Check sheet for the drawn part. Datum: minimum x, y, z corner. Units: mm. A direction names the side the tool comes from. Coordinates: 2 decimals unless noted, no trailing zeros. Write each loop counter-clockwise with the first axis right and the second up, starting at its lowest first coordinate (ties: lowest second). Pieces come first, ordered by that corner, then holes. Notation, with made-up numbers: (89.25, 45.5) -> (128.25, 45.5) arc R6 cw to (128.25, 52.5) -> close; hole circle Ø11 at (71, 89). An arc over 180 degrees is marked (long way). Answer in a Markdown table with one row per item. Add a question column.
Q1. Section check A-A, the plane x = 5. Record the boundary of the cut face in (y, z), and give its area (3 significant figures).
Q2. Section check B-B, the plane y = 15.25. Record the boundary of the cut face in (x, z).
Q3. Section check C-C, the plane z = 5. Record the boundary of the cut face in (x, y), and give its area (3 significant figures).
Q4. Gauge pin test, flat ends, axial feed: P1, Ø4, axis at x = 5, z = 5, coming from the +Y side; P2, Ø1.5, axis at y = 17, z = 15, coming from the +X side; P3, Ø1, axis at y = 14.5, z = 45.5, coming from the +X side; P4, Ø10, axis at x = 38.5, y = 6.5, coming from the +Z side. Record the tip position at first contact, or that the pin passes through.
Q5. Section check D-D, the plane x = 27.5. Record the boundary of the cut face in (y, z).
Q6. Tool access check on the marked faces 1 and 2. Record the directions out of +Z, -Z, +X, -X, +Y, -Y that give a thin tool (end or side, any length) a straight path to the whole face; none if there is none.
Q7. Thickness scan on line 1 (X direction, y = 10.75, z = 33); line 2 (Z direction, x = 39.5, y = 5.5); line 3 (X direction, y = 19.5, z = 5). Record the ranges inside material, lowest first.
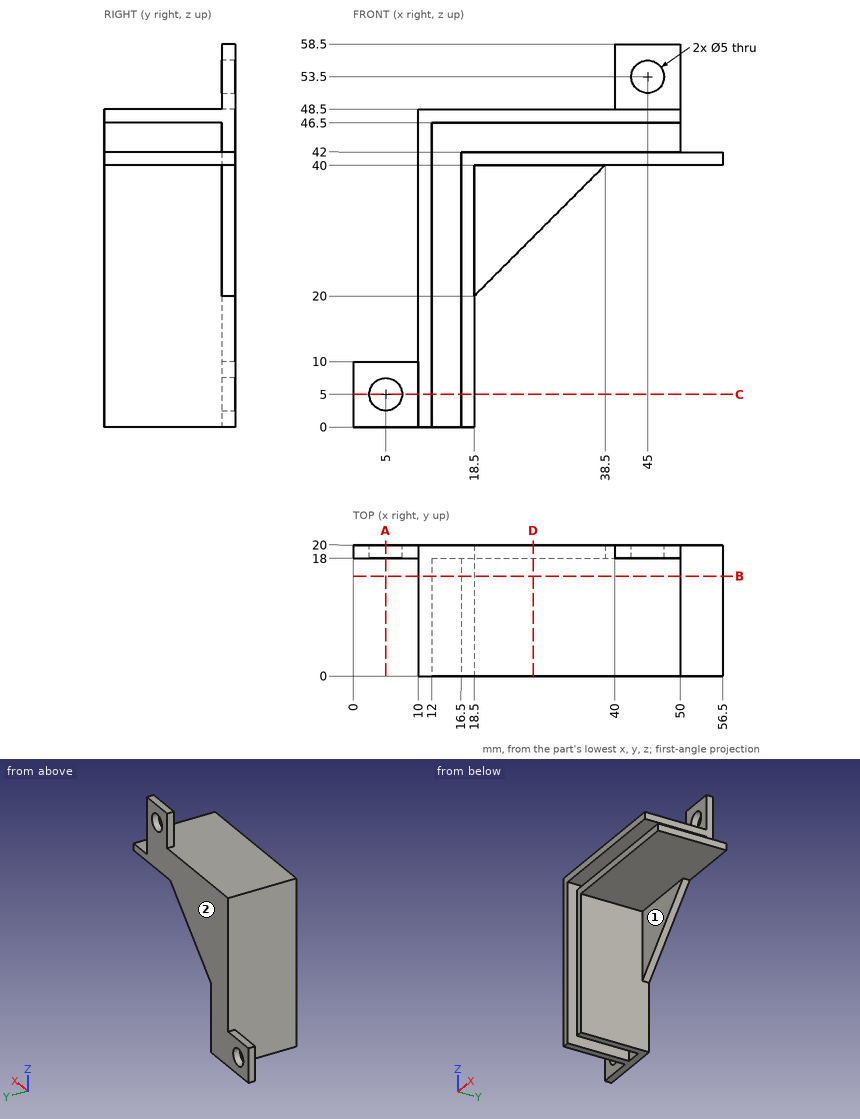
Calculated:
| question | item | result |
|---|---|---|
| 1 | outline | (18, 0) -> (20, 0) -> (20, 2.5) -> (18, 2.5) -> close; (18, 7.5) -> (20, 7.5) -> (20, 10) -> (18, 10) -> close |
| 1 | area | 10.0 mm² |
| 2 | outline | (10, 0) -> (12, 0) -> (12, 46.5) -> (50, 46.5) -> (50, 48.5) -> (10, 48.5) -> close; (16.5, 0) -> (18.5, 0) -> (18.5, 40) -> (56.5, 40) -> (56.5, 42) -> (16.5, 42) -> close |
| 3 | outline | (0, 18) -> (2.5, 18) -> (2.5, 20) -> (0, 20) -> close; (7.5, 18) -> (10, 18) -> (10, 0) -> (12, 0) -> (12, 18) -> (16.5, 18) -> (16.5, 0) -> (18.5, 0) -> (18.5, 20) -> (7.5, 20) -> close |
| 3 | area | 99.0 mm² |
| 4 | P1 | passes through |
| 4 | P2 | stops at x = 18.5 |
| 4 | P3 | stops at x = 12 |
| 4 | P4 | stops at z = 48.5 |
| 5 | outline | (0, 40) -> (18, 40) -> (18, 29) -> (20, 29) -> (20, 48.5) -> (0, 48.5) -> (0, 46.5) -> (18, 46.5) -> (18, 42) -> (0, 42) -> close |
| 6 | face 1 | -Z, +X, -Y |
| 6 | face 2 | +Z, -Z, +X, -X, +Y |
| 7 | line 1 | x = 10 to 12, 16.5 to 18.5 |
| 7 | line 2 | z = 40 to 42, 46.5 to 48.5 |
| 7 | line 3 | x = 0 to 2.5, 7.5 to 18.5 |
